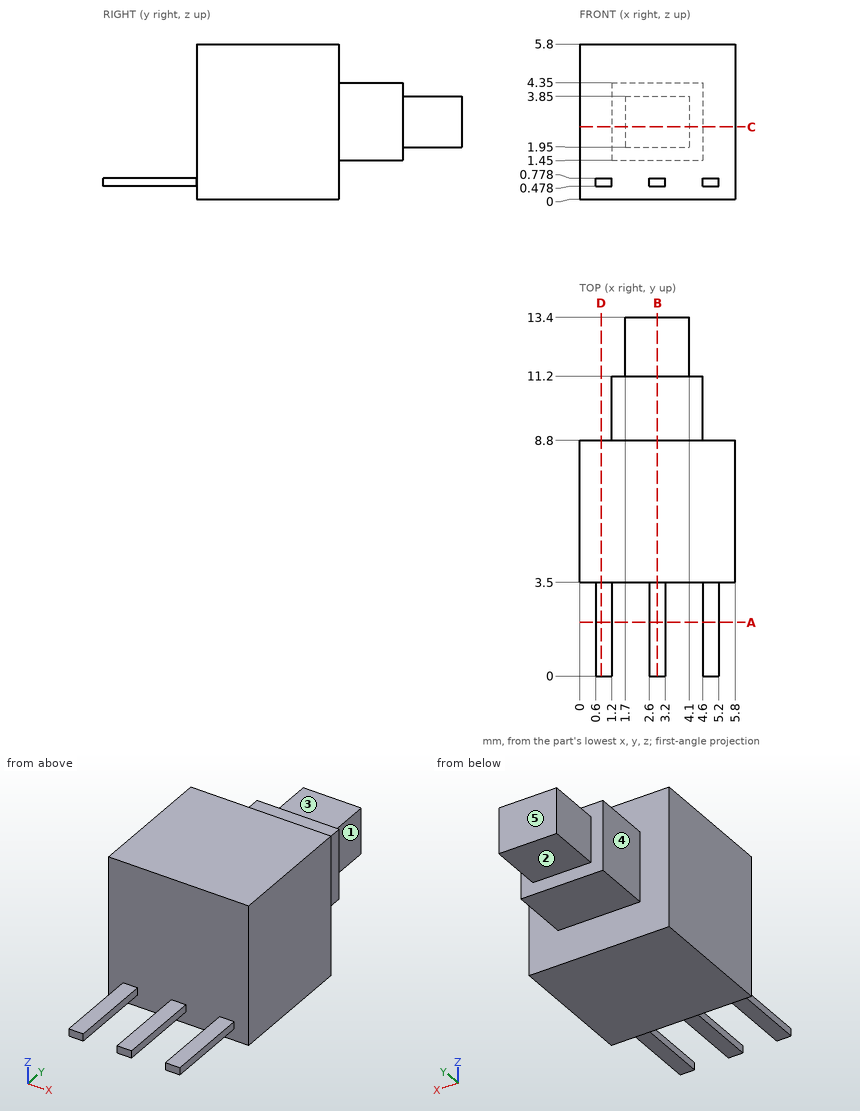
Drawing for the job (mm, zero at the part's lowest x, y, z). A direction names the side the tool comes from. Round coordinates to 2 decimals unless told otherwise and drop trailing zeros. Write each loop counter-clockwise with the first axis right and the second up, starting at its lowest first coordinate (ties: lowest second). Pieces come first, ordered by that corner, then holes. Notation, with made-up numbers: M 10,60 L 30,60 A12 cw 30,71 Z; hole C 36,74 d1. An arc over 180 degrees is marked long. One line per question, with ' | ' between items.
1. Pin check, flat tips, straight feed: pin 1 Ø1.2 at (x, y) = (3.5, 9.5) entering from +Z; pin 2 Ø0.5 at (x, y) = (5, 1.5) entering from +Z; pin 3 Ø2.5 at (x, y) = (3.5, 9.5) entering from -Z; pin 4 Ø1.1 at (x, y) = (2.5, 12.5) entering from +Z. Stop position of each tip, or through.
Working result:
pin 1: z = 4.35 | pin 2: z = 0.78 | pin 3: z = 0 | pin 4: z = 3.85
2. Cut at C-C on z = 2.7. Write the cut outline in (x, y).
Working result:
outline: M 0,3.5 L 5.8,3.5 L 5.8,8.8 L 4.6,8.8 L 4.6,11.2 L 4.1,11.2 L 4.1,13.4 L 1.7,13.4 L 1.7,11.2 L 1.2,11.2 L 1.2,8.8 L 0,8.8 Z
3. Probe L1, parallel to Y at x = 4.65, z = 0.25; L2, parallel to Y at x = 3.15, z = 3.8; L3, parallel to Z at x = 3.5, y = 10.5. List the from-to ranges inside material, lowest first. Write a range as from..to.
Working result:
L1: 3.5..8.8 | L2: 3.5..13.4 | L3: 1.45..4.35
4. Cut at D-D on x = 0.8. Write the cut outline in (y, z).
Working result:
outline: M 0,0.48 L 3.5,0.48 L 3.5,0 L 8.8,0 L 8.8,5.8 L 3.5,5.8 L 3.5,0.78 L 0,0.78 Z
5. Cut at A-A on y = 2. Write the cut outline in (x, z).
Working result:
outline: M 0.6,0.48 L 1.2,0.48 L 1.2,0.78 L 0.6,0.78 Z; M 2.6,0.48 L 3.2,0.48 L 3.2,0.78 L 2.6,0.78 Z; M 4.6,0.48 L 5.2,0.48 L 5.2,0.78 L 4.6,0.78 Z
6. Cut at B-B on x = 2.9. Write the cut outline in (y, z).
Working result:
outline: M 0,0.48 L 3.5,0.48 L 3.5,0 L 8.8,0 L 8.8,1.45 L 11.2,1.45 L 11.2,1.95 L 13.4,1.95 L 13.4,3.85 L 11.2,3.85 L 11.2,4.35 L 8.8,4.35 L 8.8,5.8 L 3.5,5.8 L 3.5,0.78 L 0,0.78 Z
7. Which spindle directions (+Z, -Z, +X, -X, +Y, -Y) get a long thin tool onto all of the face, cutting with end or side? Do the marked faces 1, 2, 3, 4 and 5. Say none if no direction does.
Working result:
face 1: +Z, -Z, +X, +Y | face 2: -Z, +X, -X, +Y | face 3: +Z, +X, -X, +Y | face 4: +Z, -Z, -X, +Y | face 5: +Z, -Z, +X, -X, +Y
